from build123d import *

# Parameters (mm, degrees)
ESQUISSE1_W             = 30
ESQUISSE1_H             = 17
EXTRUSION1_DEPTH        = 1.5
ESQUISSE2_R             = 2
ENL_V_MAT_EXTRU_1_DEPTH = 2
ESQUISSE3_W             = 1.5
ESQUISSE3_H             = 17
EXTRUSION2_DEPTH        = 23.5
ESQUISSE4_R             = 1.25
ENL_V_MAT_EXTRU_2_DEPTH = 2
EXTRUSION3_DEPTH        = 0.2
EXTRUSION3_DEPTH_BACK   = 6
ESQUISSE5_R             = 2.2
ESQUISSE5_R_2           = 1.25
CONG_1_R                = 0.5


with BuildPart() as part:
    # Esquisse1 → Extrusion1 (new body)
    with BuildSketch(Plane.XY):
        with Locations((6.051065449, -10.06674277)):
            Rectangle(ESQUISSE1_W, ESQUISSE1_H)
    extrude(amount=EXTRUSION1_DEPTH)

    # Esquisse2 → Enlèv. mat.-Extru.1 (cut)
    with BuildSketch(Plane.XY.offset(1.5)):
        with Locations((-5.463077382, -5.076163116)):
            Circle(ESQUISSE2_R)
        with Locations((4.558431294, -15.07006433)):
            Circle(ESQUISSE2_R)
    extrude(amount=-ENL_V_MAT_EXTRU_1_DEPTH, mode=Mode.SUBTRACT)

    # Esquisse3 → Extrusion2 (add)
    with BuildSketch(Plane(origin=(0, 0, 0), x_dir=(-1, 0, 0), z_dir=(0, 0, -1))):
        with Locations((-20.301065449, -10.06674277)):
            Rectangle(ESQUISSE3_W, ESQUISSE3_H)
    extrude(amount=EXTRUSION2_DEPTH)

    # Esquisse4 → Enlèv. mat.-Extru.2 (cut)
    with BuildSketch(Plane(origin=(21.051065449, 0, 0), x_dir=(0, 0, -1), z_dir=(1, 0, 0))):
        with Locations((6.5, -15.107440586)):
            Circle(ESQUISSE4_R)
        with Locations((18.5, -5.06674277)):
            Circle(ESQUISSE4_R)
    extrude(amount=-ENL_V_MAT_EXTRU_2_DEPTH, mode=Mode.SUBTRACT)

    # Esquisse5 → Extrusion3 (add, two sides: drawn at the far end of the back side and taken through both)
    # profile 1 of 2: a face of its own
    with BuildSketch(Plane(origin=(21.051065449, 0, 0), x_dir=(0, 0, -1), z_dir=(1, 0, 0)).offset(-EXTRUSION3_DEPTH_BACK)):
        with Locations(Location((6.5, -15.107440586, 0), (0, 0, 90))):
            Circle(ESQUISSE5_R)
        with Locations((6.5, -15.107440586)):
            Circle(ESQUISSE5_R_2, mode=Mode.SUBTRACT)
    # profile 2 of 2: a face of its own
    with BuildSketch(Plane(origin=(21.051065449, 0, 0), x_dir=(0, 0, -1), z_dir=(1, 0, 0)).offset(-EXTRUSION3_DEPTH_BACK)):
        with Locations(Location((18.5, -5.06674277, 0), (0, 0, 90))):
            Circle(ESQUISSE5_R)
        with Locations((18.5, -5.06674277)):
            Circle(ESQUISSE5_R_2, mode=Mode.SUBTRACT)
    extrude(amount=EXTRUSION3_DEPTH + EXTRUSION3_DEPTH_BACK)

    # Congé1
    cong_1_edges = [part.edges().sort_by_distance(p)[0] for p in [
        (20.301065449, -18.56674277, -23.5),
        (20.301065449, -1.56674277, -23.5),
        (-8.948934551, -18.56674277, 0.75),
        (-8.948934551, -1.56674277, 0.75),
    ]]
    fillet(cong_1_edges, radius=CONG_1_R)


solid = part.part
Verification items for the finished model (mm, model axes). A direction names the side the tool comes from. Give positions to 0.01 mm unless a question says otherwise; leave off trailing zeros. Loops run counter-clockwise (first coordinate to the right, second up) from the corner with the lowest first, then second, coordinate; pieces in that order, holes last.
1) Sectioned sample at A-A, the plane z = -18.5. Enter the section's corners in (x, y).
2) Set-up check for faces 5 (the flat face through (15.051, -3.6, -18.5)), 6 (the cylindrical face through (17.27, -17.305, -6.403)), 7 (the flat face through (10.7, -1.567, 0.2)): record each of +Z, -Z, +X, -X, +Y, -Y from which the full face is reachable in a straight line by a thin tool's end or side.
3) Thickness scan on line 1 along Y through (x, z) = (19, -18.5); line 2 along Z through (x, y) = (2.5, -16.5); line 3 along Z through (x, y) = (16, -14.25). Record the ranges inside material, lowest first.
4) Sectioned sample at B-B, the plane y = -4.5. Enter the section's corners in (x, z).
5) Sectioned sample at C-C, the plane x = 17. Enter the section's corners in (y, z), then the cut area to 3 significant figures.
6) Depth check by flat-ended pin: pin 1 Ø1.5 at (x, y) = (12.5, -8.5) entering from -Z; pin 2 Ø1 at (y, z) = (-12, -5.5) entering from -X; pin 3 Ø3 at (x, y) = (-5.46, -5.08) entering from -Z; pin 4 Ø1.3 at (y, z) = (-4, -17.5) entering from -X. Enter the tip coordinate at first touch or a pass-through.
7) Draft check along X on faces 1 (the flat face through (21.051, -10, -11)), 2 (the cylindrical face through (4.12, -17.02, 0.76)), 3 (the cylindrical face through (-4.54, -6.85, 0.76)), 4 (the flat face through (-8.949, -10, 1)). Enter one of: pulls with the +X half, pulls with the -X half, needs draft (parallel to the pull), parting line crosses it, or undercut.
8) Sectioned sample at D-D, the plane y = -9.75. Enter the section's corners in (x, z).
Answers:
1. outline: (15.05, -7.27) - (19.55, -7.27) - (19.55, -18.57) - (21.05, -18.57) - (21.05, -7.27) - (21.25, -7.27) - (21.25, -6.32) - (15.05, -6.32) - close; (15.05, -3.82) - (21.25, -3.82) - (21.25, -2.87) - (21.05, -2.87) - (21.05, -1.57) - (19.55, -1.57) - (19.55, -2.87) - (15.05, -2.87) - close
2. face 5: -Z, -X, +Y, -Y
2. face 6: -X
2. face 7: +Z, -Z, +X, -X, +Y
3. line 1: y = -7.27 to -6.32, -3.82 to -2.87
3. line 2: z = 0 to 1.5
3. line 3: z = -8.53 to -7.41, -5.59 to -4.47, 0 to 1.5
4. outline: (-8.95, 0) - (-7.38, 0) - (-7.38, 1.5) - (-8.95, 1.5) - close; (-3.55, 0) - (19.55, 0) - (19.55, -16.37) - (15.05, -16.37) - (15.05, -17.39) - (21.25, -17.39) - (21.25, -16.37) - (21.05, -16.37) - (21.05, 1.5) - (-3.55, 1.5) - close; (15.05, -20.63) - (19.55, -20.63) - (19.55, -23.5) - (21.05, -23.5) - (21.05, -20.63) - (21.25, -20.63) - (21.25, -19.61) - (15.05, -19.61) - close
5. outline: (-18.57, 0) - (-1.57, 0) - (-1.57, 1.5) - (-18.57, 1.5) - close; circle Ø4.4 at (-15.11, -6.5); circle Ø4.4 at (-5.07, -18.5); hole circle Ø2.5 at (-15.11, -6.5); hole circle Ø2.5 at (-5.07, -18.5)
5. area: 46.1 mm2
6. pin 1: stops at z = 0
6. pin 2: stops at x = 19.55
6. pin 3: passes through
6. pin 4: stops at x = 15.05
7. face 1: pulls with the +X half
7. face 2: undercut
7. face 3: undercut
7. face 4: pulls with the -X half
8. outline: (-8.95, 0) - (19.55, 0) - (19.55, -23.5) - (21.05, -23.5) - (21.05, 1.5) - (-8.95, 1.5) - close
